```python
from build123d import *

# Parameters (mm, degrees)
REVOLVE8_ANGLE      = 180
SKETCH5_W           = 2.85
SKETCH5_H           = 4.85
BOSS_EXTRUDE1_DEPTH = 2
SKETCH6_W           = 3
SKETCH6_H           = 5
CUT_EXTRUDE1_DEPTH  = 2
FILLET1_R           = 1


with BuildPart() as part:
    # Sketch3 → Revolve8 (revolve)
    with BuildSketch(Plane.XY):
        with BuildLine():
            Line((-29.128306284, 11.200453936), (-37.660231074, 74.93674596))
            Line((-37.660231074, 74.93674596), (-39.127877823, 74.93674596))
            Line((-39.127877823, 74.93674596), (-39.127877823, -13.799546064))
            Line((-39.127877823, -13.799546064), (-26.361565762, -13.799546064))
            ThreePointArc((-26.361565762, -13.799546064), (-27.930281109, -3.066483557), (-23.370793287, 6.77580121))
            Line((-23.370793287, 6.77580121), (-23.370793287, 11.200453936))
            Line((-23.370793287, 11.200453936), (-29.128306284, 11.200453936))
        make_face()
    revolve(axis=Axis((-9.127877823, 95.858464184, 0), (0, -1, 0)), revolution_arc=REVOLVE8_ANGLE)

    # Sketch5 → Boss-Extrude1 (add)
    with BuildSketch(Plane.XY):
        with Locations((16.447122177, 13.700453936)):
            Rectangle(SKETCH5_W, SKETCH5_H)
    extrude(amount=BOSS_EXTRUDE1_DEPTH)

    # Sketch6 → Cut-Extrude1 (cut)
    with BuildSketch(Plane.XY):
        with Locations((-34.627877823, 13.700453936)):
            Rectangle(SKETCH6_W, SKETCH6_H)
    extrude(amount=-CUT_EXTRUDE1_DEPTH, mode=Mode.SUBTRACT)

    # Fillet1
    fillet1_edges = [part.edges().sort_by_distance(p)[0] for p in [
        (-9.127877823, -13.799546064, -17.23368794),
    ]]
    fillet(fillet1_edges, radius=FILLET1_R)


solid = part.part
```
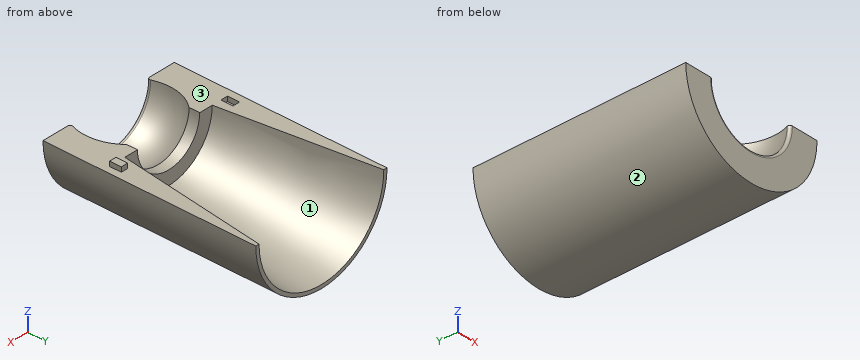
Geometry check sheet. Reference: the model listing, model coordinates, mm. Face numbers are marked on the shaded views. Coordinates: 2 decimals unless noted, no trailing zeros. Write each loop counter-clockwise with the first axis right and the second up, starting at its lowest first coordinate (ties: lowest second). Pieces come first, ordered by that corner, then holes. Notation, with made-up numbers: M 42,-38.5 L 84,-38.5 A19 cw 84,-22.5 Z; hole C 80.5,28 d11. An arc over 180 degrees is marked long. Use one line per item in the form item = value. Start each with the question number.
1) Section check B-B on y = -3. Enter the section's corners in (x, z).
2) Section check A-A on y = 40.5. Enter the section's corners in (x, z), and give its area (3 significant figures).
3) Thickness scan on probe 1 along Y at (x, z) = (10, -5); probe 2 along X at (y, z) = (53, -11); probe 3 along X at (y, z) = (17, -3). Record the ranges inside material, lowest first. Write a range as from..to.
4) Go/stop test with flat-tipped pins: pin 1 Ø8 at (x, y) = (-8, 25) entering from -Z; pin 2 Ø3 at (x, y) = (-24, 35.5) entering from +Z; pin 3 Ø4 at (x, y) = (-31, 55) entering from -Z. Record where each tip stops, or that it passes through.
5) Release check for a two-part mould opening along X. For the marked faces 1, 2 and 3 record: pulls with the +X half, pulls with the -X half, needs draft (parallel to the pull), parting line crosses it, or undercut.
Responses:
q1.outline = M -39.13,0 A30 ccw 20.87,0 L 9.66,0 A18.79 cw -27.92,0 Z
q2.outline = M -39.13,0 A30 ccw 20.87,0 L 14.79,0 A23.92 cw -33.05,0 Z
q2.area = 515 mm2
q3.probe_1 = -13.8..11.2
q3.probe_2 = -37.04..-32.24, 13.98..18.78
q3.probe_3 = -38.98..-29.69, 11.43..20.72
q4.pin_1 = -30
q4.pin_2 = -16.49
q4.pin_3 = -22.47
q5.face_1 = undercut
q5.face_2 = parting line crosses it
q5.face_3 = needs draft
